Part model, mm, in its own coordinate system. A direction names the side the tool comes from. Round coordinates to 2 decimals unless told otherwise and drop trailing zeros. Order: outer loops, then holes, each group sorted by start corner. A loop starts at its lowest first (then second) coordinate and runs counter-clockwise, first axis right, second up. Notation, with made-up numbers: (-14.75, 65) -> (3.25, 65) arc R20 ccw to (3.25, 96) -> close; hole circle Ø3 at (35.25, -3.75). An arc over 180 degrees is marked (long way). Return JSON: item names as keys, results as strings. Group by question number.
Autodesk Inventor part; units mm, degrees
ref_plane "YZ Plane" through (0, 0, 0) normal (1, 0, 0) x (0, 1, 0)
ref_plane "XZ Plane" through (0, 0, 0) normal (0, 1, 0) x (-1, 0, 0)
ref_plane "XY Plane" through (0, 0, 0) normal (0, 0, 1) x (1, 0, 0)
sketch "Sketch1" plane through (0, 0, 0) normal (0, 1, 0) x (-1, 0, 0)
  circle A0 centre (0, 9.5) radius 1.5
  circle A1 centre (0, -9.5) radius 1.5
  line L0 (-3, 6) -> (3, 6)
  line L1 (3, 6) -> (3, -6)
  line L2 (3, -6) -> (-3, -6)
  line L3 (-3, -6) -> (-3, 6)
  line L4 (-3, 6) -> (3, -6) construction
  line L5 (3, 6) -> (-3, -6) construction
  line L6 (3, 12.2) -> (-3, 12.2)
  line L7 (-3, 12.2) -> (-3, -12.2)
  line L8 (-3, -12.2) -> (3, -12.2)
  line L9 (3, -12.2) -> (3, 12.2)
  line L10 (3, 12.2) -> (-3, -12.2) construction
  line L11 (-3, 12.2) -> (3, -12.2) construction
  line L12 (0, 12.2) -> (5, 12.2)
  line L13 (0, 12.2) -> (-5, 12.2)
  line L14 (-5, 12.2) -> (-5, -19.8)
  line L15 (-5, -19.8) -> (5, -19.8)
  line L16 (5, -19.8) -> (5, 12.2)
  line L17 (5, -19.8) -> (-0.01, -19.8)
  line L18 (4.99, -13.83) -> (-5.01, -13.83)
  line L19 (-5.01, -13.83) -> (-5.01, -19.83)
  line L20 (-5.01, -19.83) -> (4.99, -19.83)
  line L21 (4.99, -19.83) -> (4.99, -13.83)
  line L22 (4.99, -13.83) -> (-5.01, -19.83) construction
  line L23 (-5.01, -13.83) -> (4.99, -19.83) construction
  line L24 (3, 6) -> (3, 1.5)
  line L25 (3, 1.5) -> (-3, 1.5)
  line L26 (-3, 6) -> (3, 6)
  line L27 (-3, 6) -> (-3, 1.5)
  line L28 (3, -6) -> (3, -1.5)
  line L29 (3, -1.5) -> (-3, -1.5)
  line L30 (-3, -1.5) -> (-3, -6)
  line L31 (-3, -6) -> (3, -6)
  line L32 (-0.01, -16.83) -> (-0.01, -19.8)
  point P0 (0, 0)
  point P1 (0, 0)
  point P2 (0, -30.9776)
  point P3 (-5, -13.83)
  point P4 (-5, -19.33)
  point P5 (4.99, -19.8)
  dimension "d0" = 3
  dimension "d1" = 3
  dimension "d2" = 19
  dimension "d3" = 6
  dimension "d4" = 12
  dimension "d5" = 3.5
  dimension "d6" = 3.5
  dimension "d7" = 6
  dimension "d8" = 24.4
  dimension "d11" = 5
  dimension "d12" = 5
  dimension "d13" = 32
  dimension "d14" = 90
  dimension "d15" = 10
  dimension "d16" = 5.01
  dimension "d18" = 10
  dimension "d19" = 6
  dimension "d20" = 4.5
  dimension "d21" = 4.5
extrude "Extrusion5" add sketch "Sketch1" against normal blind 1.6 contours A0 | A1 | L7 L6 L9 L0 | L0 L1 L25 L3 | L3 L7 L8 L9 L1 L12 L16 L15 L21 L18 L14 L13 | L25 L1 L29 L3 | L29 L1 L2 L3 | L2 L9 L8 L7 | L18 L21 L15 L14
extrude "Extrusion6" cut sketch "Sketch1" along normal mid plane 10 contours A0
extrude "Extrusion7" cut sketch "Sketch1" along normal mid plane 10 contours A1
extrude "Extrusion8" add sketch "Sketch1" along normal blind 3 contours L7 L6 L9 L0
extrude "Extrusion9" add sketch "Sketch1" along normal blind 3 contours L2 L9 L8 L7
extrude "Extrusion10" add sketch "Sketch1" against normal blind 9 contours L18 L21 L15 L14
extrude "Extrusion11" add sketch "Sketch1" along normal blind 3 contours L25 L1 L29 L3
extrude "Extrusion12" add sketch "Sketch1" along normal blind 11 contours L0 L1 L25 L3
extrude "Extrusion13" add sketch "Sketch1" along normal blind 11 contours L29 L1 L2 L3
sketch "Sketch2" plane through (-3, 3, -1.5) normal (0, 0, 1) x (1, 0, 0)
  line L0 (0, 8) -> (6, 8)
  line L1 (0, 8) -> (2.25, 8)
  line L2 (0, -3) -> (6, -3)
  line L3 (2.25, 8) -> (2.25, 3)
  line L4 (2.25, 3) -> (3.75, 3)
  line L5 (3.75, 3) -> (3.75, 8)
  line L6 (3.75, 8) -> (6, 8)
  line L7 (2.25, 8) -> (3.75, 8)
  point P0 (3, -3)
  dimension "d48" = 2.25
  dimension "d49" = 5
  dimension "d50" = 1.5
extrude "Extrusion14" cut sketch "Sketch2" against normal blind 2
sketch "Sketch3" plane through (3, 3, 1.5) normal (0, 0, -1) x (-1, 0, 0)
  line L0 (0, 8) -> (6, 8)
  line L1 (0, 8) -> (2.25, 8)
  line L2 (2.25, 8) -> (2.25, 3)
  line L3 (3.75, 3) -> (3.75, 8)
  line L4 (2.25, 3) -> (3.75, 3)
  line L5 (3.75, 3) -> (3.75, 8)
  line L6 (3.75, 8) -> (2.25, 8)
  point P0 (3, -3)
  dimension "d53" = 2.25
  dimension "d54" = 5
  dimension "d55" = 1.5
extrude "Extrusion15" cut sketch "Sketch3" against normal blind 2
properties part number "photointerrupter"
(1) Saw through at A-A, the plane z = 9.5. List the corners of the cut face in (x, y).
(2) Pin check, flat tips, straight feed: P1, Ø5, axis at x = 0.5, y = 6, coming from the -Z side; P2, Ø0.6, axis at y = 9, z = 2.5, coming from the +X side; P3, Ø0.8, axis at x = 0, z = -2.5, coming from the +Y side; P4, Ø2.5, axis at x = 0, z = -9.5, coming from the +Y side. Stop position of each tip, or through.
(3) Mould opens along X. For faces 5 (the flat face through (5, -1, -11)), 6 (the flat face through (0.75, 8, -2)), 7 (the flat face through (0.75, 9, 2)), 8 (the flat face through (0, -9, -17)) say: pulls with the +X half, pulls with the -X half, needs draft (parallel to the pull), parting line crosses it, or undercut.
(4) Tool access for faces 1 (the flat face through (1, 7, -1.5)), 2 (the flat face through (-3, 2, 0)), 3 (the flat face through (0, 3, -7.7)), 4 (the flat face through (-0.75, 9, -2)): list every direction of +Z, -Z, +X, -X, +Y, -Y with a clear straight run to the whole face (end or side of a thin tool).
(5) Probe L1, parallel to Z at x = 0, y = 0.9; L2, parallel to Z at x = 2, y = 6.75; L3, parallel to Z at x = 0.5, y = 1.75. List the from-to ranges inside material, lowest first. Write a range as [from, to].
(6) Saw through at C-C, the plane y = 7.25. List the corners of the cut face in (x, z), and give its area (3 significant figures).
(7) Saw through at D-D, the plane y = -0.5. List the corners of the cut face in (x, z), and give its area (3 significant figures).
(8) Saw through at B-B, the plane x = 0. List the corners of the cut face in (y, z), and give its area (3 significant figures).
Results are:
{
 "1": {"outline": "(-5, -1.6) -> (-1.5, -1.6) -> (-1.5, 3) -> (-3, 3) -> (-3, 0) -> (-5, 0) -> close; (1.5, -1.6) -> (5, -1.6) -> (5, 0) -> (3, 0) -> (3, 3) -> (1.5, 3) -> close"},
 "2": {"P1": "stops at z = -6", "P2": "stops at x = 3", "P3": "stops at y = 6", "P4": "passes through"},
 "3": {"face 5": "pulls with the +X half", "face 6": "undercut", "face 7": "undercut", "face 8": "needs draft"},
 "4": {"face 1": "+X, -X, +Y", "face 2": "+Z, -Z, -X, +Y", "face 3": "-Z, +X, -X, +Y", "face 4": "+Y"},
 "5": {"L1": "z = [-12.2, -11], [-8, 8], [11, 12.2]", "L2": "z = [-6, -1.5], [1.5, 6]", "L3": "z = [-12.2, -10.91], [-8.09, 8.09], [10.91, 12.2]"},
 "6": {"outline": "(-3, -6) -> (3, -6) -> (3, -1.5) -> (0.75, -1.5) -> (0.75, -3.5) -> (-0.75, -3.5) -> (-0.75, -1.5) -> (-3, -1.5) -> close; (-3, 1.5) -> (-0.75, 1.5) -> (-0.75, 3.5) -> (0.75, 3.5) -> (0.75, 1.5) -> (3, 1.5) -> (3, 6) -> (-3, 6) -> close", "area": "48.0 mm^2"},
 "7": {"outline": "(-5, -19.8) -> (5, -19.8) -> (5, 12.2) -> (-5, 12.2) -> close; hole circle Ø3 at (0, -9.5); hole circle Ø3 at (0, 9.5)", "area": "306 mm^2"},
 "8": {"outline": "(-9, -19.8) -> (0, -19.8) -> (0, -12.2) -> (3, -12.2) -> (3, -11) -> (-1.6, -11) -> (-1.6, -13.83) -> (-9, -13.83) -> close; (-1.6, -8) -> (3, -8) -> (3, -6) -> (11, -6) -> (11, -3.5) -> (6, -3.5) -> (6, -1.5) -> (3, -1.5) -> (3, 1.5) -> (6, 1.5) -> (6, 3.5) -> (11, 3.5) -> (11, 6) -> (3, 6) -> (3, 8) -> (-1.6, 8) -> close; (-1.6, 11) -> (3, 11) -> (3, 12.2) -> (-1.6, 12.2) -> close", "area": "193 mm^2"}
}
